Input: dimensioned drawing with shaded views. Units: mm. Origin: part minimum x, y, z. Give positions to 0.01 mm unless a question says otherwise; leave off trailing zeros. Write each loop counter-clockwise with the first axis right and the second up, starting at its lowest first coordinate (ties: lowest second). Pieces come first, ordered by that corner, then holes. Notation, with made-up numbers: (86.25, -12.5) -> (104.25, -12.5) arc R24 ccw to (104.25, 22.5) -> close; hole circle Ø1 at (-11.75, 57.25). An arc over 180 degrees is marked (long way). Answer as a JSON object with one key per item and string values. Group by question number.
(1) Draft query along X for the marked faces 1, 2 and 3. Return one class per face: +X half, -X half, draft (parallel to the pull), parting line (faces both ways), or undercut.
(2) Section query A-A on y = 13. Output: boundary loops of the cut face in (x, z) (1 decimal).
(3) Contact query for flat-ended pins moving along their axis: pin 1 Ø12 at (y, z) = (3.5, 28.5) entering from +X; pin 2 Ø10 at (y, z) = (6.5, 30) entering from +X; pin 3 Ø1.5 at (y, z) = (7, 8.5) entering from +X (1 decimal). Output: stop coordinate, or through.
(4) Material intervals for probe 1 along X at (y, z) = (6.75, 17.5) (1 decimal); probe 2 along Z at (x, y) = (29, 12.5) (1 decimal); probe 3 along X at (y, z) = (2.75, 26.5) (1 decimal), sorted ascending.
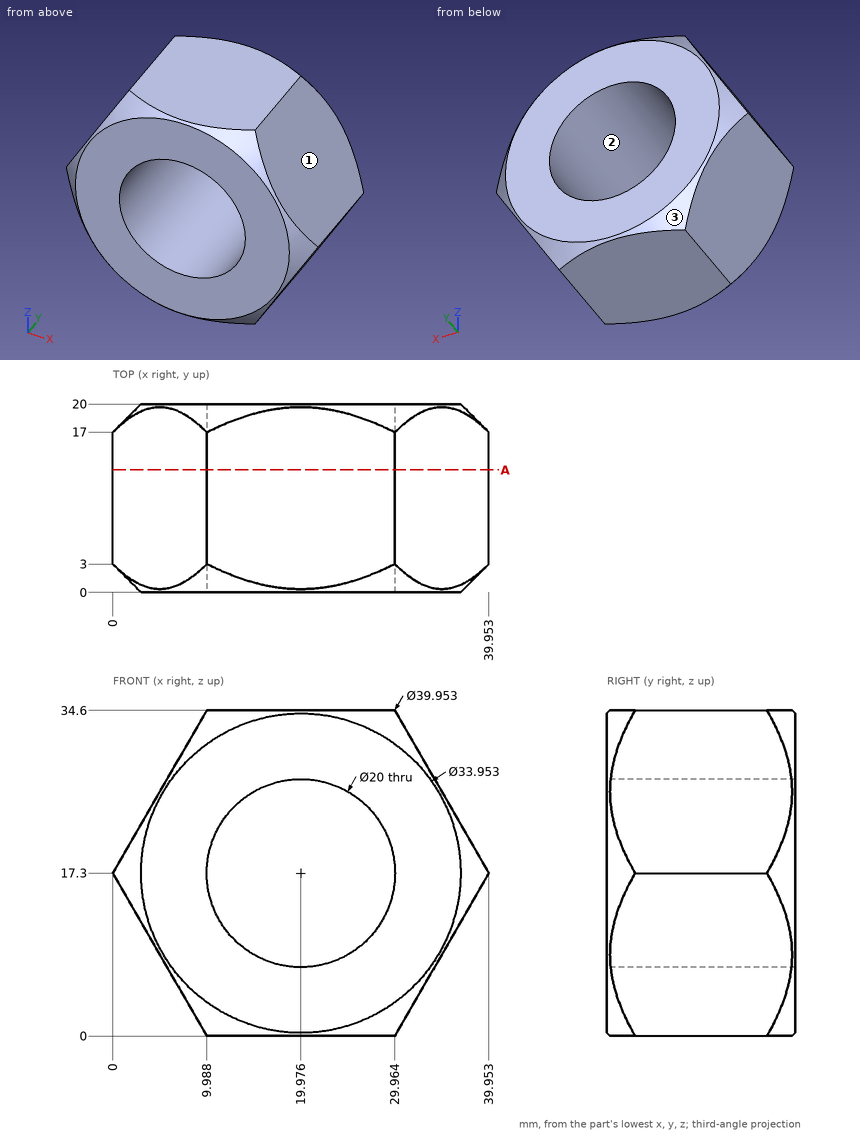
Answer list:
{
 "1": {"face 1": "+X half", "face 2": "undercut", "face 3": "parting line"},
 "2": {"outline": "(0, 17.3) -> (10, 0) -> (30, 0) -> (40, 17.3) -> (30, 34.6) -> (10, 34.6) -> close; hole circle Ø20 at (20, 17.3)"},
 "3": {"pin 1": "x = 36.95", "pin 2": "x = 35.51", "pin 3": "x = 35.3"},
 "4": {"probe 1": "0.1 to 10, 30 to 39.8", "probe 2": "0 to 13, 21.6 to 34.6", "probe 3": "5.3 to 16.1, 23.9 to 34.6"}
}
